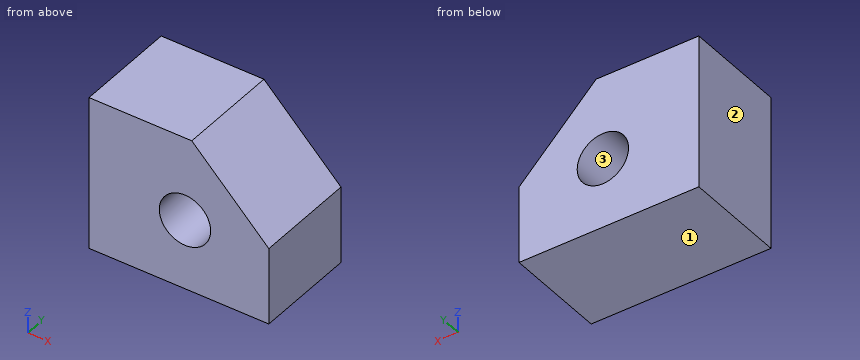
from build123d import *

# Parameters (mm, degrees)
F0_W     = 88.9
F0_H     = 76.2
F1_DEPTH = 50.8
F2_SIZE  = 38.1
F3_R     = 12.7
F4_DEPTH = 50.8


with BuildPart() as f1:
    # F0 (on Front) → F1 (new body)
    with BuildSketch(Plane.XZ):
        with Locations((-2.997909, 3.463231)):
            Rectangle(F0_W, F0_H)
    extrude(amount=F1_DEPTH)

    # F2
    f2_edges = [f1.edges().sort_by_distance(p)[0] for p in [
        (41.452091, -25.4, 41.563231),
    ]]
    chamfer(f2_edges, length=F2_SIZE)

    # F3 (on face) → F4 (cut)
    with BuildSketch(Plane.XZ.offset(50.8)):
        Circle(F3_R)
    extrude(amount=-F4_DEPTH, mode=Mode.SUBTRACT)


solid = f1.part
Verification items for the finished model (mm, model axes). Face numbers are marked on the shaded views. Coordinates: 2 decimals unless noted, no trailing zeros. Loops run counter-clockwise (first coordinate to the right, second up) from the corner with the lowest first, then second, coordinate; pieces in that order, holes last. Notation, with made-up numbers: (81.25, -11) -> (107.25, -11) arc R4 cw to (107.25, -7) -> close; hole circle Ø10 at (66.5, 7). An arc over 180 degrees is marked (long way). Answer as CSV lines item,"result".
1) Depth check by flat-ended pin: pin 1 (3 mm diameter, centred on y = -21, z = 18, fed in from +X); pin 2 (6 mm diameter, centred on y = -31.5, z = 27, fed in from +X). Enter the tip coordinate at first touch or a pass-through.
Found:
pin 1,"stops at x = 28.42"
pin 2,"stops at x = 20.92"
2) Cross-section at D-D, the plane x = 35. Record the cut outline in (y, z).
Found:
outline,"(-50.8, -34.64) -> (0, -34.64) -> (0, 9.92) -> (-50.8, 9.92) -> close"
3) Cross-section at A-A, the plane x = 0. Record the cut outline in (y, z), then the cut area to 3 significant figures.
Found:
outline,"(-50.8, -34.64) -> (0, -34.64) -> (0, -12.7) -> (-50.8, -12.7) -> close; (-50.8, 12.7) -> (0, 12.7) -> (0, 41.56) -> (-50.8, 41.56) -> close"
area,"2,580 mm2"
4) Thickness scan on L1, parallel to Z at x = 0, y = -36.5; L2, parallel to X at y = -19, z = -10; L3, parallel to X at y = -30, z = -11.5. Record the ranges inside material, lowest first. Write a range as from..to.
Found:
L1,"z = -34.64..-12.7, 12.7..41.56"
L2,"x = -47.45..-7.83, 7.83..41.45"
L3,"x = -47.45..-5.39, 5.39..41.45"
5) Cross-section at B-B, the plane y = -28. Record the cut outline in (x, z).
Found:
outline,"(-47.45, -34.64) -> (41.45, -34.64) -> (41.45, 3.46) -> (3.35, 41.56) -> (-47.45, 41.56) -> close; hole circle Ø25.4 at (0, 0)"
6) Cross-section at C-C, the plane z = -7. Record the cut outline in (x, y), then the cut area to 3 significant figures.
Found:
outline,"(-47.45, -50.8) -> (-10.6, -50.8) -> (-10.6, 0) -> (-47.45, 0) -> close; (10.6, -50.8) -> (41.45, -50.8) -> (41.45, 0) -> (10.6, 0) -> close"
area,"3,440 mm2"
7) Release check for a two-part mould opening along Z. For the marked faces 1, 2 and 3 record: +Z half, -Z half, draft (parallel to the pull), parting line (faces both ways), or undercut.
Found:
face 1,"-Z half"
face 2,"draft"
face 3,"undercut"
